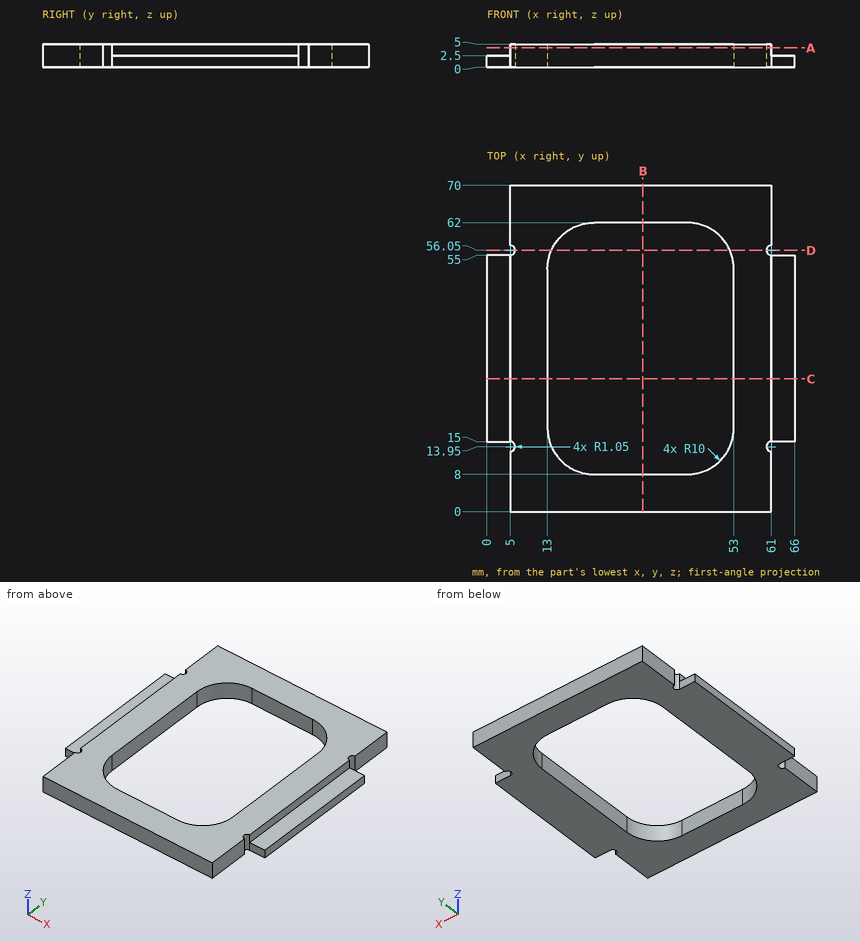
Here's the drawing with two shaded views (mm, measured from the low corner). I have some questions. Give positions to 0.01 mm unless a question says otherwise; leave off trailing zeros. Write each loop counter-clockwise with the first axis right and the second up, starting at its lowest first coordinate (ties: lowest second). Pieces come first, ordered by that corner, then holes. Notation, with made-up numbers: (-20.5, 53.5) - (19.5, 53.5) arc R19 ccw to (19.5, 74.5) - close; hole circle Ø10 at (88, 52.5). An arc over 180 degrees is marked (long way). One line per item, written item: value. Start each with the question number.
Item 1: Please list where these lines run through material, in increasing order: line 1 (X direction, y = 48, z = 4); line 2 (X direction, y = 28, z = 1.9); line 3 (Y direction, x = 40, z = 3.2). Write a range as from..to.
Item 2: I'm going to push flat-ended pins straight in: pin 1 (0.8 mm diameter, centred on x = 62.5, z = 1, fed in from -Y); pin 2 (2.5 mm diameter, centred on y = 64, z = 2.5, fed in from +X); pin 3 (2.5 mm diameter, centred on x = 2.5, y = 41.5, fed in from +Z). Where does each tip first touch, or does it pass through?
Item 3: Imagine slicing it at C-C, the plane y = 28.5. List the corners of the cut face in (x, z) for me.
Item 4: Imagine slicing it at D-D, the plane y = 56.05. List the corners of the cut face in (x, z) for me.
Item 5: Imagine slicing it at B-B, the plane x = 33.5. List the corners of the cut face in (y, z) for me, and give its area (3 significant figures).
Item 6: Imagine slicing it at A-A, the plane z = 4.15. List the corners of the cut face in (x, y) for me.
Geometry says:
1. line 1: 5..13, 53..61
1. line 2: 0..13, 53..66
1. line 3: 0..8, 62..70
2. pin 1: y = 15
2. pin 2: x = 61
2. pin 3: z = 2.5
3. outline: (0, 0) - (13, 0) - (13, 5) - (5, 5) - (5, 2.5) - (0, 2.5) - close; (53, 0) - (66, 0) - (66, 2.5) - (61, 2.5) - (61, 5) - (53, 5) - close
4. outline: (6.05, 0) - (13.86, 0) - (13.86, 5) - (6.05, 5) - close; (52.14, 0) - (59.95, 0) - (59.95, 5) - (52.14, 5) - close
5. outline: (0, 0) - (8, 0) - (8, 5) - (0, 5) - close; (62, 0) - (70, 0) - (70, 5) - (62, 5) - close
5. area: 80.0 mm^2
6. outline: (5, 0) - (61, 0) - (61, 12.9) arc R1.05 cw to (61, 15) - (61, 55) arc R1.05 cw to (61, 57.1) - (61, 70) - (5, 70) - (5, 57.1) arc R1.05 cw to (5, 55) - (5, 15) arc R1.05 cw to (5, 12.9) - close; hole (13, 18) arc R10 ccw to (23, 8) - (43, 8) arc R10 ccw to (53, 18) - (53, 52) arc R10 ccw to (43, 62) - (23, 62) arc R10 ccw to (13, 52) - close
